The model under review builds one solid part; all positions refer to its coordinate system, in mm. Face numbers are marked on the shaded views. A direction names the side the tool comes from. Coordinates: 2 decimals unless noted, no trailing zeros. Order: outer loops, then holes, each group sorted by start corner. A loop starts at its lowest first (then second) coordinate and runs counter-clockwise, first axis right, second up. Notation, with made-up numbers: (10.5, 25.5) -> (62.5, 25.5) arc R7 ccw to (62.5, 32.5) -> close; hole circle Ø2 at (1, -10.75). An arc over 180 degrees is marked (long way). Use one line per item in the form item = value.
from build123d import *

# Parameters (mm, degrees)
F1_DEPTH      = 1.5875
F1_DEPTH_BACK = 1.5875
F2_DEPTH      = 6.35
F2_DEPTH_BACK = 6.35
F4_DEPTH      = 3.175
F7_DEPTH      = 9.525
F8_W          = 3.175
F8_H          = 9.525
F9_DEPTH      = 6.35
F10_R         = 14.2875
F11_DEPTH     = 3.175


with BuildPart() as f1:
    # F0 (on Front) → F1 (new body, two sides)
    with BuildSketch(Plane.XZ) as f1_sk:
        with BuildLine():
            Line((6.5154837304, 17.901144426), (0, 0))
            ThreePointArc((0, 0), (31.4472391318, 28.1249079907), (69.85, 45.593945062))
            Line((69.85, 45.593945062), (53.975, 51.371972531))
            Line((53.975, 51.371972531), (6.5154837304, 17.901144426))
        make_face()
    extrude(amount=-F1_DEPTH)
    extrude(f1_sk.sketch, amount=F1_DEPTH_BACK)


with BuildPart() as f1b:
    # F0 (on Front) → F1, piece 2 (new body, two sides)
    with BuildSketch(Plane.XZ) as f1_2_sk:
        with BuildLine():
            Line((13.0309674607, 35.8022888519), (8.4178990072, 23.1279874415))
            Line((8.4178990072, 23.1279874415), (50.3413574439, 52.6945102634))
            Line((50.3413574439, 52.6945102634), (38.1, 57.15))
            ThreePointArc((38.1, 57.15), (28.0500865293, 43.558427019), (13.0309674607, 35.8022888519))
        make_face()
    extrude(amount=-F1_DEPTH)
    extrude(f1_2_sk.sketch, amount=F1_DEPTH_BACK)


with BuildPart() as f2:
    # F0 (on Front) → F2 (new body, two sides)
    with BuildSketch(Plane.XZ) as f2_sk:
        Polygon((8.4178990072, 23.1279874415), (6.5154837304, 17.901144426), (53.975, 51.371972531), (50.3413574439, 52.6945102634), align=None)
    extrude(amount=-F2_DEPTH)
    extrude(f2_sk.sketch, amount=F2_DEPTH_BACK)

    # F3 (on face) → F4 (cut)
    with BuildSketch(Plane(origin=(-6.2670410681, 0, 8.8862676656), x_dir=(0.8172112207, 0, 0.5763382867), z_dir=(0.5763382867, 0, -0.8172112207))):
        with BuildLine():
            Line((73.7166102717, 6.35), (15.6416413214, 6.35))
            ThreePointArc((15.6416413214, 6.35), (44.6791257965, 1.5875), (73.7166102717, 6.35))
        make_face()
        with BuildLine():
            ThreePointArc((73.7166102717, -6.35), (44.6791257965, -1.5875), (15.6416413214, -6.35))
            Line((15.6416413214, -6.35), (73.7166102717, -6.35))
        make_face()
    extrude(amount=-F4_DEPTH, mode=Mode.SUBTRACT)


with BuildPart() as f1b_1:
    add(f1b.part)

    # F5: union F2, F1
    add(f2.part)
    add(f1.part)

    # F6 (on face) → F7 (join)
    with BuildSketch(Plane(origin=(0, 0, 0), x_dir=(0, -1, 0), z_dir=(-0.9396926208, 0, 0.3420201433))):
        Polygon((1.5875, 33.7373950786), (-1.5875, 33.7373950786), (-1.5875, 24.6122901573), (-1.5875, 19.05), (-1.5875, 9.9248950786), (1.5875, 9.9248950786), (1.5875, 19.05), (1.5875, 24.6122901573), align=None)
    extrude(amount=F7_DEPTH)

    # F8 (on face) → F9 (cut)
    with BuildSketch(Plane(origin=(0, 0, 0), x_dir=(0, -1, 0), z_dir=(-0.9396926208, 0, 0.3420201433))):
        with Locations((0, 28.9748950786)):
            Rectangle(F8_W, F8_H)
        with Locations((0, 14.6873950786)):
            Rectangle(F8_W, F8_H)
    extrude(amount=F9_DEPTH, mode=Mode.SUBTRACT)

    # F10 (on face) → F11 (join)
    with BuildSketch(Plane(origin=(0, 0, 0), x_dir=(0, -1, 0), z_dir=(-0.9396926208, 0, 0.3420201433))):
        with Locations((-0.0234540593, 21.8311450786)):
            Circle(F10_R)
        Polygon((-1.5875, 33.7373950786), (1.5875, 33.7373950786), (1.5875, 24.6122901573), (1.5875, 19.05), (1.5875, 9.9248950786), (-1.5875, 9.9248950786), (-1.5875, 19.05), (-1.5875, 24.6122901573), align=None, mode=Mode.SUBTRACT)
        Polygon((1.5875, 24.6122901573), (1.5875, 33.7373950786), (-1.5875, 33.7373950786), (-1.5875, 24.6122901573), (-1.5875, 19.05), (-1.5875, 9.9248950786), (1.5875, 9.9248950786), (1.5875, 19.05), align=None)
    extrude(amount=F11_DEPTH)


solid = f1b_1.part
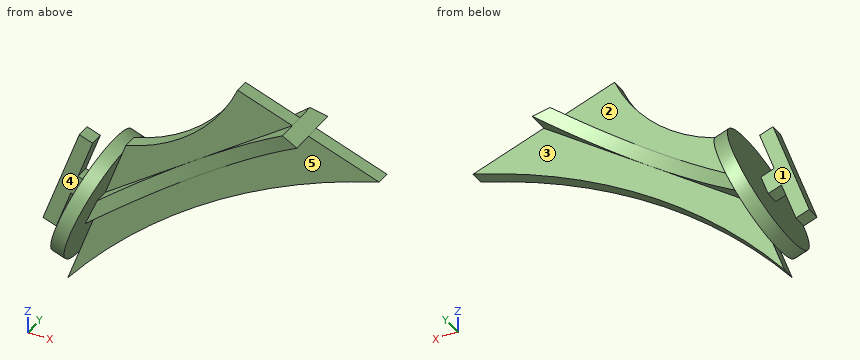
Item 1: Clearance check with flat-ended pins moving along their axes: pin 1 (12 mm diameter, centred on x = 51.5, y = 1.5, fed in from -Z); pin 2 (3.5 mm diameter, centred on x = 0.5, z = 27, fed in from -Y); pin 3 (5 mm diameter, centred on y = -8, z = 7, fed in from +X). State where each tip first meets the part, or that it passes through.
Results found:
pin_1 = 36.18
pin_2 = -1.59
pin_3 = 3.46
Item 2: Tool access review of the marked faces 3, 4 and 5: name each direction out of +Z, -Z, +X, -X, +Y, -Y from which nothing blocks a thin tool from reaching the whole face with its end or side.
Results found:
face_3 = -Z, +X, +Y
face_4 = +Z, -X, -Y
face_5 = -Z, +X, -Y
Item 3: Draft analysis for pull direction X (two halves, no side actions). For the marked faces 1 and 2, state which applies: released by +X, released by -X, zero draft, split by the parting line, or undercut.
Results found:
face_1 = zero draft
face_2 = undercut
Item 4: We need section A-A (y = 0). Write out the cut boundary in (x, z) (3 decimals), plus the area to 3 significant figures.
Results found:
outline = (-5.556, 12.584) -> (-2.573, 11.498) -> (0.685, 20.449) -> (3.669, 19.363) -> (-0.403, 8.175) -> (2.58, 7.089) -> (0, 0) arc R139.877 cw to (69.85, 45.594) -> (38.1, 57.15) arc R37.28 cw to (13.031, 35.802) -> (12.353, 33.94) -> (9.37, 35.026) -> (5.298, 23.838) -> (2.314, 24.924) -> (5.572, 33.875) -> (2.588, 34.961) -> close
area = 1,180 mm²
Item 5: We need section B-B (y = 11). Write out the cut boundary in (x, z).
Results found:
outline = (1.36, 13.01) -> (4.34, 11.92) -> (10.59, 29.11) -> (7.61, 30.19) -> close
Item 6: To check wall thickness, follow L1, parallel to Y at x = 29, z = 42.5; L2, parallel to X at y = -5.5, z = 11; L3, parallel to Z at x = 16, y = 0.5. State the ranges of each line that lie inside material, in increasing order. Write a range as from..to.
Results found:
L1 = -1.59..1.59
L2 = 0.62..4
L3 = 16.44..36.69
Item 7: We need section C-C (y = -9.25). Write out the cut boundary in (x, z).
Results found:
outline = (0.77, 11.39) -> (3.75, 10.3) -> (11.18, 30.73) -> (8.2, 31.81) -> close
